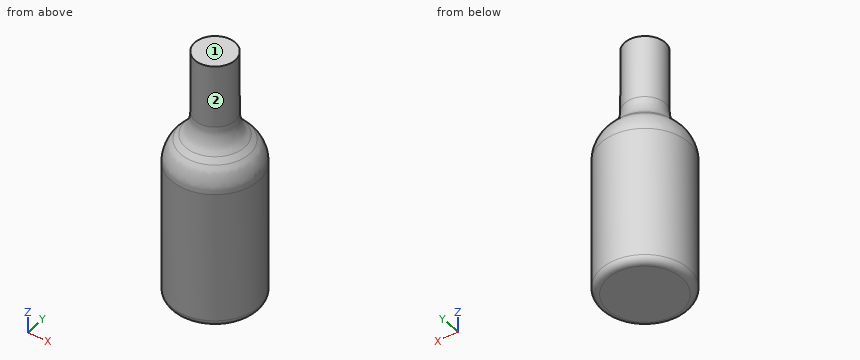
```python
from build123d import *

# Parameters (mm, degrees)
F2_R = 5.08
F3_R = 25.4


with BuildPart() as f1:
    # F0 (on Front) → F1 (revolve)
    with BuildSketch(Plane.XZ):
        Polygon((15.24, 95.25), (0, 95.25), (0, -95.25), (33.02, -95.25), (33.02, 19.05), (15.24, 37.494287), align=None)
    revolve(axis=Axis((0, 0, 2.313137), (0, 0, -1)))

    # F2
    f2_edges = [f1.edges().sort_by_distance(p)[0] for p in [
        (-33.02, 0, -95.25),
    ]]
    fillet(f2_edges, radius=F2_R)

    # F3
    f3_edges = [f1.edges().sort_by_distance(p)[0] for p in [
        (-33.02, 0, 19.05),
        (-15.24, 0, 37.494287),
    ]]
    fillet(f3_edges, radius=F3_R)


solid = f1.part
```
Geometry check sheet. Reference: the model listing, model coordinates, mm. Face numbers are marked on the shaded views. A direction names the side the tool comes from. Give positions to 0.01 mm unless a question says otherwise; leave off trailing zeros. Loops run counter-clockwise (first coordinate to the right, second up) from the corner with the lowest first, then second, coordinate; pieces in that order, holes last. Notation, with made-up numbers: (42.5, 82.25) - (57.5, 82.25) arc R38 ccw to (57.5, 121.25) - close; hole circle Ø9 at (70, 6.5). An arc over 180 degrees is marked (long way). Use CSV: the item, a comma, the result in double quotes. Start each with the question number.
Q1. Scan lines: probe 1 along Y at (x, z) = (6.5, -60.5); probe 2 along X at (y, z) = (6, -82); probe 3 along X at (y, z) = (-11.5, -33). Record each from-to range of solid material in increasing order. Write a range as from..to.
Q2. Section check A-A, the plane z = -74. Record the cut outline in (x, y), and give its area (3 significant figures).
Q3. Go/stop test with flat-tipped pins: pin 1 Ø12 at (x, z) = (16, 24.5) entering from -Y; pin 2 Ø6 at (x, z) = (-22.5, 5.5) entering from -Y; pin 3 Ø2 at (x, z) = (7.5, 51.5) entering from +Y. Record where each tip stops, or that it passes through.
Q4. Access from +Z, -Z, +X, -X, +Y, -Y to the whole of each face (thin tool, end or side, straight path). Record for the marked faces 1 and 2.
Findings below:
1,probe 1,"y = -32.37..32.37"
1,probe 2,"x = -32.47..32.47"
1,probe 3,"x = -30.95..30.95"
2,outline,"circle Ø66.04 at (0, 0)"
2,area,"3,430 mm^2"
3,pin 1,"stops at y = -27.94"
3,pin 2,"stops at y = -26.65"
3,pin 3,"stops at y = 13.78"
4,face 1,"+Z, +X, -X, +Y, -Y"
4,face 2,"+Z"
